from build123d import *

# Parameters (mm, degrees)
F0_W             = 1190
F0_H             = 630
F1_DEPTH         = 20
F4_DEPTH         = 20.001
F4_COPIES2_COUNT = 2
F4_COPIES2_PITCH = 779.860552
F5_DEPTH         = 20.001
F7_R             = 17.515
F7_R_2           = 10.05
F8_DEPTH         = 20.001
F11_R            = 2.5
F12_DEPTH        = 20.001
F12_COPIES_COUNT = 4
F9_W             = 1190
F9_H             = 242.437693119
F13_DEPTH        = 20.001


# Not quite as in the source:
# - a pattern or mirror of a feature is missing from the dataset's text; its kind, count and spacing are read off the source's solid


with BuildPart() as f1:
    # F0 (on Top) → F1 (new body)
    with BuildSketch(Plane.XY):
        Rectangle(F0_W, F0_H)
    extrude(amount=F1_DEPTH)

    # F3 (on face) → F4 (cut, through all)
    with BuildSketch(Plane.XY.offset(20)):
        with BuildLine():
            Line((-323.2, 255), (-323.2, 193.2))
            ThreePointArc((-323.2, 193.2), (-319.1, 189.1), (-315, 193.2))
            Line((-315, 193.2), (-315, 255))
            ThreePointArc((-315, 255), (-319.1, 259.1), (-323.2, 255))
        make_face()
    f4 = extrude(amount=-F4_DEPTH, mode=Mode.SUBTRACT)

    # F4_copies: F4 across plane
    add(f4.mirror(Plane(origin=(0, 0, 0), x_dir=(0, 0, 1), z_dir=(1, 0, 0))), mode=Mode.SUBTRACT)

    # F4_copies1: F4 across plane
    add(f4.mirror(Plane(origin=(0, 0, 0), x_dir=(0, 0, -1), z_dir=(0, -1, 0))), mode=Mode.SUBTRACT)

    # F4_copies2: F4 ×2
    with Locations(*[Vector(0.818351433, -0.5747181327, 0) * (i * F4_COPIES2_PITCH) for i in range(1, F4_COPIES2_COUNT)]):
        add(f4, mode=Mode.SUBTRACT)

    # F3 (on face) → F5 (cut, through all)
    with BuildSketch(Plane.XY.offset(20)):
        with BuildLine():
            Line((-398, -8.5), (-315, -8.5))
            ThreePointArc((-315, -8.5), (-306.5, 0), (-315, 8.5))
            Line((-315, 8.5), (-398, 8.5))
            ThreePointArc((-398, 8.5), (-406.5, 0), (-398, -8.5))
        make_face()
    f5 = extrude(amount=-F5_DEPTH, mode=Mode.SUBTRACT)

    # F5_copies: F5 across plane
    add(f5.mirror(Plane(origin=(0, 0, 0), x_dir=(0, 0, 1), z_dir=(1, 0, 0))), mode=Mode.SUBTRACT)

    # F7 (on face) → F8 (cut, through all)
    with BuildSketch(Plane.XY.offset(20)):
        with Locations((-50, -225)):
            Circle(F7_R)
        with Locations((50, -225)):
            Circle(F7_R_2)
    extrude(amount=-F8_DEPTH, mode=Mode.SUBTRACT)

    # F11 (on face) → F12 (cut, through all)
    with BuildSketch(Plane.XY.offset(20)):
        with Locations((-308, 308)):
            Circle(F11_R)
        with Locations((-184.8, 308)):
            Circle(F11_R)
        with Locations((-61.6, 308)):
            Circle(F11_R)
        with Locations((61.6, 308)):
            Circle(F11_R)
        with Locations((184.8, 308)):
            Circle(F11_R)
        with Locations((308, 308)):
            Circle(F11_R)
    f12 = extrude(amount=-F12_DEPTH, mode=Mode.SUBTRACT)

    # F12_copies: F12 ×4 about axis
    f12_copies_axis = Axis((0, 0, 0), (0, 0, 1))
    for i in range(1, F12_COPIES_COUNT):
        add(f12.rotate(f12_copies_axis, i * 360 / F12_COPIES_COUNT), mode=Mode.SUBTRACT)

    # F9 (on face) → F13 (cut, through all)
    with BuildSketch(Plane.XY.offset(20)):
        with Locations((0, 436.2188465595)):
            Rectangle(F9_W, F9_H)
    extrude(amount=-F13_DEPTH, mode=Mode.SUBTRACT)


solid = f1.part
CAD build for the part. Positions are in the model's coordinates, mm. Give positions to 0.01 mm unless a question says otherwise; leave off trailing zeros. Put each result on its own line as item: value. Start each with the question number.
(1) Flat gauge pin, fed straight in: pin 1 Ø4 at (x, y) = (-184.8, 308) entering from -Z. Where does the tip first touch, or does it go through?
(2) Probe L1, parallel to Y at x = 184.8, z = 9.75; L2, parallel to X at y = -61.6, z = 5.25; L3, parallel to X at y = -255.5, z = 6.25. List the from-to ranges inside material, lowest first.
(3) Mould opens along X. For faces 1 (the face through (-8, 4, 20)), 2 (the face through (-53.797, -242.099, 10.14)) say: +X half, -X half, draft (parallel to the pull), parting line (faces both ways), or undercut.
Response values:
1. pin 1: passes through
2. L1: y = -315 to -310.5, -305.5 to 305.5, 310.5 to 315
2. L2: x = -595 to -310.5, -305.5 to 305.5, 310.5 to 595
2. L3: x = -595 to -323.17, -315.03 to 315.03, 323.17 to 595
3. face 1: draft
3. face 2: undercut
